from build123d import *

# Parameters (mm, degrees)
SKETCH1_R           = 9.9
BOSS_EXTRUDE1_DEPTH = 7
SKETCH1_3_R         = 12
BOSS_EXTRUDE2_DEPTH = 1
SKETCH1_4_R         = 1.65
CUT_EXTRUDE1_DEPTH  = 11
CUT_EXTRUDE2_DEPTH  = 4


with BuildPart() as part:
    # Sketch1 → Boss-Extrude1 (new body)
    with BuildSketch(Plane(origin=(0, 0, 0), x_dir=(1, 0, 0), z_dir=(0, 1, 0))):
        with Locations((-1.873325665, 1.210998997)):
            Circle(SKETCH1_R)
    extrude(amount=-BOSS_EXTRUDE1_DEPTH)

    # Sketch1<3> → Boss-Extrude2 (add)
    with BuildSketch(Plane(origin=(0, 0, 0), x_dir=(1, 0, 0), z_dir=(0, 1, 0))):
        with Locations((-1.873325665, 1.210998997)):
            Circle(SKETCH1_3_R)
    extrude(amount=-BOSS_EXTRUDE2_DEPTH)

    # Sketch1<4> → Cut-Extrude1 (cut)
    with BuildSketch(Plane(origin=(0, 0, 0), x_dir=(1, 0, 0), z_dir=(0, 1, 0))):
        with Locations((-0.93043169, 7.320486504)):
            Circle(SKETCH1_4_R)
        with Locations((-0.93043169, -4.621555184)):
            Circle(SKETCH1_4_R)
        with Locations((-7.873325665, 1.210998997)):
            Circle(SKETCH1_4_R)
        with Locations((4.126674335, 1.210998997)):
            Circle(SKETCH1_4_R)
    extrude(amount=-CUT_EXTRUDE1_DEPTH, mode=Mode.SUBTRACT)

    # Sketch1<5> → Cut-Extrude2 (cut)
    with BuildSketch(Plane(origin=(0, 0, 0), x_dir=(1, 0, 0), z_dir=(0, 1, 0))):
        Polygon((-6.100068619, -1.56128516), (-4.585828635, 1.360542568), (-6.359085682, 4.132826725), (-9.646582711, 3.983283154), (-11.160822695, 1.061455426), (-9.387565648, -1.710828731), align=None)
        Polygon((6.021818673, -1.47943367), (7.404229541, 1.507025804), (5.509085203, 4.197458471), (2.231529997, 3.901431664), (0.849119129, 0.91497219), (2.744263467, -1.775460477), align=None)
    extrude(amount=-CUT_EXTRUDE2_DEPTH, mode=Mode.SUBTRACT)


solid = part.part
Model file for the job. Use its own axes, mm. A direction names the side the tool comes from. Give positions to 0.01 mm unless a question says otherwise; leave off trailing zeros. Loops run counter-clockwise (first coordinate to the right, second up) from the corner with the lowest first, then second, coordinate; pieces in that order, holes last.
1) Flat gauge pins, fed straight in: pin 1 Ø4 at (x, y) = (-8.5, -5) entering from -Z; pin 2 Ø1.5 at (y, z) = (-4.5, -2) entering from -X; pin 3 Ø1.8 at (x, z) = (4.5, -2.5) entering from +Y. Where does each tip first touch, or does it go through?
2) Pull direction Z, two halves, no side cores. Call faces 1 (the flat face through (-7.98, -1.97, -4.06)), 2 (the flat face through (-2, 0, -1)), 3 (the cylindrical face through (-4.5, -0.5, 10.5)), 4 (the flat face through (6, -4, 0)): +Z half, -Z half, draft (parallel to the pull), parting line (faces both ways), or undercut.
3) Tool access for faces 5 (the flat face through (6.7, -1.97, 0.01)), 6 (the flat face through (-6.4, -1, -10.2)), 7 (the cylindrical face through (5.7, -5.48, -1.71)): list every direction of +Z, -Z, +X, -X, +Y, -Y with a clear straight run to the whole face (end or side of a thin tool).
4) Saw through at C-C (x = -3). Write the cut outline in (y, z), plus the area to 3 significant figures.
5) Wall check: line 1 (Z direction, x = -1.5, y = -4.75); line 2 (X direction, y = -0.25, z = -3.75) (3 decimals); line 3 (X direction, y = -1.5, z = -1.25). Give the ranges that are in metal, low to high.
6) Saw through at A-A (x = 4). Write the cut outline in (y, z), plus the area to 3 significant figures.
7) Saw through at B-B (y = -3.25). Write the cut outline in (x, z), plus the area to 3 significant figures.
8) Saw through at D-D (x = -10.75). Write the cut outline in (y, z), plus the area to 3 significant figures.
Answer block:
1. pin 1: stops at z = -9.96
1. pin 2: stops at x = -11.77
1. pin 3: stops at y = -4
2. face 1: undercut
2. face 2: draft
2. face 3: parting line
2. face 4: undercut
3. face 5: +Y
3. face 6: -Y
3. face 7: +Y, -Y
4. outline: (-7, -11.05) - (-1, -11.05) - (-1, -13.16) - (0, -13.16) - (0, 10.74) - (-1, 10.74) - (-1, 8.62) - (-7, 8.62) - close
4. area: 142 mm2
5. line 1: z = -11.1 to -8.87, -5.77 to 3.07, 6.17 to 8.68
5. line 2: x = -13.602 to -9.767, -6.114 to 2.161, 5.824 to 9.855
5. line 3: x = -11.77 to -11.06, -4.64 to 1, 7.29 to 8.03
6. outline: (-7, -9.18) - (-1, -9.18) - (-1, -11.68) - (0, -11.68) - (0, -4.06) - (-4, -4.06) - (-4, -2.86) - (-7, -2.86) - close; (-7, 0.43) - (-4, 0.43) - (-4, 1.66) - (0, 1.66) - (0, 9.25) - (-1, 9.25) - (-1, 6.76) - (-7, 6.76) - close
6. area: 83.8 mm2
7. outline: circle Ø19.8 at (-1.87, -1.21); hole (-11.16, -1.06) - (-9.65, -3.98) - (-6.36, -4.13) - (-4.59, -1.36) - (-6.1, 1.56) - (-9.39, 1.71) - close; hole circle Ø3.3 at (-0.93, -7.32); hole circle Ø3.3 at (-0.93, 4.62); hole (0.85, -0.91) - (2.23, -3.9) - (5.51, -4.2) - (7.4, -1.51) - (6.02, 1.48) - (2.74, 1.78) - close
7. area: 235 mm2
8. outline: (-7, -5.59) - (-1, -5.59) - (-1, -9.29) - (0, -9.29) - (0, -1.85) - (-4, -1.85) - (-4, -0.42) - (0, -0.42) - (0, 6.86) - (-1, 6.86) - (-1, 3.17) - (-7, 3.17) - close
8. area: 63.0 mm2
